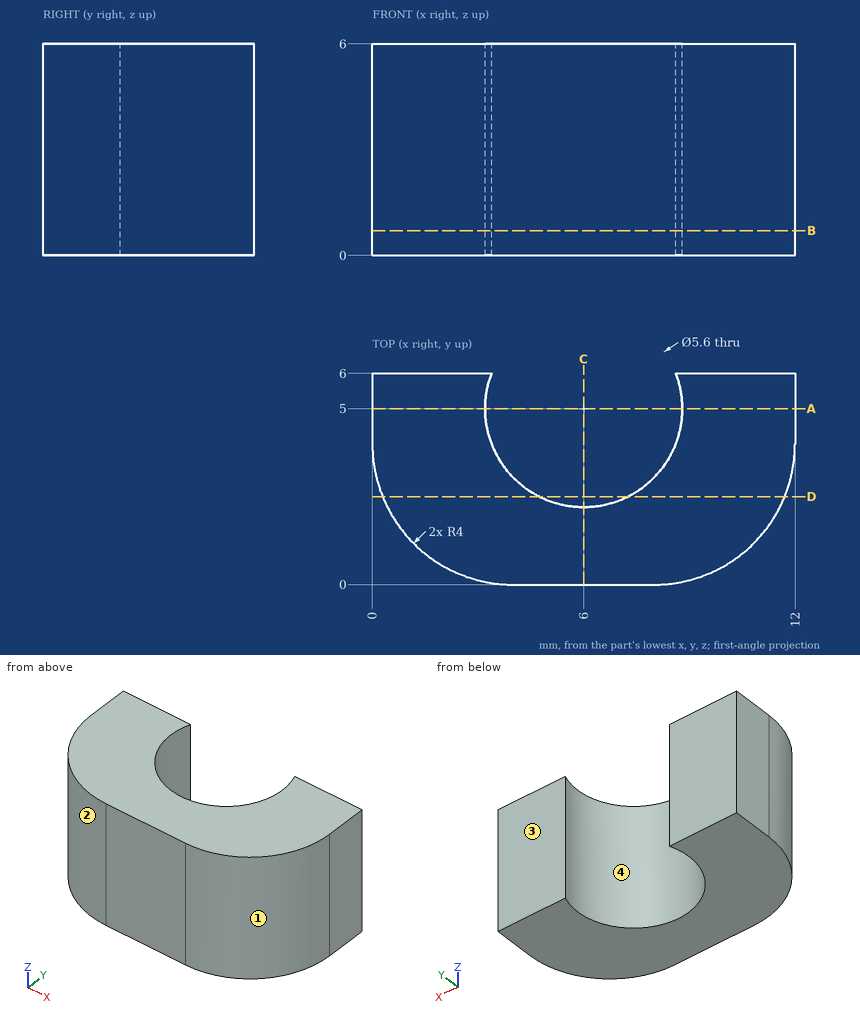
For this review, use the dimensioned drawing (mm, ordinates from the lowest corner) and the shaded views. Give positions to 0.01 mm unless a question says otherwise; leave off trailing zeros. Write each loop counter-clockwise with the first axis right and the second up, starting at its lowest first coordinate (ties: lowest second). Pieces come first, ordered by that corner, then holes. Notation, with made-up numbers: M 26.25,-9.75 L 64.25,-9.75 A19 cw 64.25,-1.75 Z; hole C 4.5,80 d5. An arc over 180 degrees is marked long. Answer as a JSON object with one key per item and string values. Group by question number.
Item 1: Draft analysis for pull direction X (two halves, no side actions). For the marked faces 1, 2, 3 and 4, state which applies: +X half, -X half, draft (parallel to the pull), parting line (faces both ways), or undercut.
Item 2: Consider section A-A on y = 5. Write out the cut boundary in (x, z).
Item 3: For pin 1 Ø1.5 at (x, z) = (4, 2) entering from +Y, flat-tipped, find the tip position at first contact; note if it passes through.
Item 4: Consider section D-D on y = 2.5. Write out the cut boundary in (x, z).
Item 5: For probe 1 along X at (y, z) = (5, 2.6); probe 2 along Y at (x, z) = (6, 3.75); probe 3 along X at (y, z) = (4.25, 2.85), list the stretches that pass through material, from the lowest coordinate up. Write a range as [from, to].
Item 6: Consider section C-C on x = 6. Write out the cut boundary in (y, z), plus the area to 3 significant figures.
Item 7: Consider section B-B on z = 0.7. Write out the cut boundary in (x, y).
Check result:
{
 "1": {"face 1": "+X half", "face 2": "-X half", "face 3": "draft", "face 4": "undercut"},
 "2": {"outline": "M 0,0 L 3.2,0 L 3.2,6 L 0,6 Z; M 8.8,0 L 12,0 L 12,6 L 8.8,6 Z"},
 "3": {"pin 1": "stops at y = 6"},
 "4": {"outline": "M 0.29,0 L 4.74,0 L 4.74,6 L 0.29,6 Z; M 7.26,0 L 11.71,0 L 11.71,6 L 7.26,6 Z"},
 "5": {"probe 1": "x = [0, 3.2], [8.8, 12]", "probe 2": "y = [0, 2.2]", "probe 3": "x = [0, 3.3], [8.7, 12]"},
 "6": {"outline": "M 0,0 L 2.2,0 L 2.2,6 L 0,6 Z", "area": "13.2 mm^2"},
 "7": {"outline": "M 0,4 A4 ccw 4,0 L 8,0 A4 ccw 12,4 L 12,6 L 8.62,6 A2.8 cw long 3.38,6 L 0,6 Z"}
}
